```python
from build123d import *

# Parameters (mm, degrees)
F0_R     = 19.05
F1_DEPTH = 25.4
F0_W     = 154.669017
F0_H     = 90.966787
F0_R_2   = 6.35
F0_R_3   = 7.532176
F2_DEPTH = 12.7
F3_D     = 25.4


with BuildPart() as f1:
    # F0 (on Front) → F1 (new body)
    with BuildSketch(Plane.XZ):
        with Locations((-18.855859, 0)):
            Circle(F0_R)
    extrude(amount=F1_DEPTH)

    # F0 (on Front) → F2 (join)
    with BuildSketch(Plane.XZ):
        with Locations((-20.002499, -1.783664)):
            Rectangle(F0_W, F0_H)
        with Locations((-85.171133, -33.938222)):
            Circle(F0_R_2, mode=Mode.SUBTRACT)
        with Locations((43.452755, -33.938222)):
            Circle(F0_R_3, mode=Mode.SUBTRACT)
        with Locations((-85.171133, 31.799983)):
            Circle(F0_R_2, mode=Mode.SUBTRACT)
        with Locations((-18.855859, 0)):
            Circle(F0_R, mode=Mode.SUBTRACT)
        with Locations((43.452755, 31.799983)):
            Circle(F0_R_2, mode=Mode.SUBTRACT)
    extrude(amount=F2_DEPTH)

    # F3 (through all)
    with Locations(Plane(origin=(0, 0, 0), x_dir=(1, 0, 0), z_dir=(0, 1, 0))):
        with Locations((-18.855859, 0)):
            Hole(F3_D / 2)


solid = f1.part
```
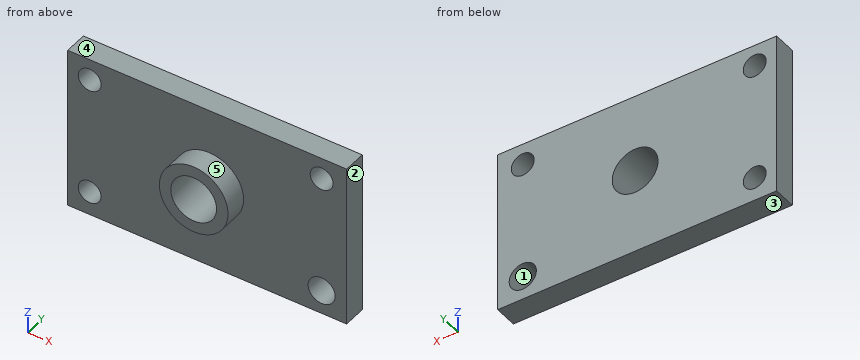
Work out the finished part from the listing and answer in its coordinate system (mm). Face numbers are marked on the shaded views. A direction names the side the tool comes from. Give positions to 0.01 mm unless a question says otherwise; leave off trailing zeros. Order: outer loops, then holes, each group sorted by start corner. A loop starts at its lowest first (then second) coordinate and runs counter-clockwise, first axis right, second up. Notation, with made-up numbers: M -15.75,52 L 34.25,52 A16 ccw 34.25,71 Z; hole C 81,-2 d8. An arc over 180 degrees is marked long. Return JSON: item names as keys, results as strings.
1) Each of these flat-tipped pins is pushed along its axis until it touches: pin 1 (12 mm diameter, centred on x = -20, z = -17.5, fed in from +Y); pin 2 (5 mm diameter, centred on x = 17.5, z = 15, fed in from -Y); pin 3 (20.5 mm diameter, centred on x = -18.86, z = 0, fed in from -Y). Where does it stop, or does it pass through?
Resolved:
{"pin 1": "y = 0", "pin 2": "y = -12.7", "pin 3": "through"}
2) Section D-D, the plane y = -9.25 is taken. Write down the section's boundary in (x, z), plus the area to 3 significant figures.
Resolved:
{"outline": "M -97.34,-47.27 L 57.33,-47.27 L 57.33,43.7 L -97.34,43.7 Z; hole C -85.17,-33.94 d12.7; hole C -85.17,31.8 d12.7; hole C -18.86,0 d25.4; hole C 43.45,-33.94 d15.06; hole C 43.45,31.8 d12.7", "area": "13,000 mm^2"}
3) Section C-C, the plane z = -37 is taken. Write down the section's boundary in (x, y).
Resolved:
{"outline": "M -97.34,-12.7 L -90.73,-12.7 L -90.73,0 L -97.34,0 Z; M -79.61,-12.7 L 36.57,-12.7 L 36.57,0 L -79.61,0 Z; M 50.33,-12.7 L 57.33,-12.7 L 57.33,0 L 50.33,0 Z"}
4) Straight lines are drawn through the part: line 1 along X through (y, z) = (-10, 26); line 2 along X through (y, z) = (-1, 30.5); line 3 along Y through (x, z) = (29, 2). For each, find the intervals that lie inside material, in ascending order. Write a range as [from, to].
Resolved:
{"line 1": "[-97.34, -87.76], [-82.59, 40.87], [46.04, 57.33]", "line 2": "[-97.34, -91.39], [-78.96, 37.24], [49.67, 57.33]", "line 3": "[-12.7, 0]"}
5) Section A-A, the plane z = 0 is taken. Write down the section's boundary in (x, y).
Resolved:
{"outline": "M -97.34,-12.7 L -37.91,-12.7 L -37.91,-25.4 L -31.56,-25.4 L -31.56,0 L -97.34,0 Z; M -6.16,-25.4 L 0.19,-25.4 L 0.19,-12.7 L 57.33,-12.7 L 57.33,0 L -6.16,0 Z"}
6) A tool of negligible diameter and unlimited length cuts with its end or side. For the marked faces 4 and 5, from which of +Z, -Z, +X, -X, +Y, -Y can it reach the whole face along a straight path? Write none if from no direction.
Resolved:
{"face 4": "+Z, +X, -X, +Y, -Y", "face 5": "-Y"}
7) For a pull along X with two mould halves and no side action, classify the marked faces 1, 2 and 3 as +X half, -X half, draft (parallel to the pull), parting line (faces both ways), or undercut.
Resolved:
{"face 1": "undercut", "face 2": "+X half", "face 3": "draft"}
8) Section B-B, the plane x = -21 is taken. Write down the section's boundary in (y, z), plus the area to 3 significant figures.
Resolved:
{"outline": "M -25.4,-18.93 L -12.7,-18.93 L -12.7,-47.27 L 0,-47.27 L 0,-12.52 L -25.4,-12.52 Z; M -25.4,12.52 L 0,12.52 L 0,43.7 L -12.7,43.7 L -12.7,18.93 L -25.4,18.93 Z", "area": "1,000 mm^2"}
